```python
from build123d import *

# Parameters (mm, degrees)
SKETCH007_R  = 4
PAD003_DEPTH = 20
SKETCH001_R  = 4
PAD004_DEPTH = 32
PAD006_DEPTH = 4
PAD001_DEPTH = 4
SKETCH_R     = 4.1
PAD_DEPTH    = 80
PAD008_DEPTH = 10


with BuildPart() as rodhole01:
    # Sketch007 → Pad003 (new body)
    with BuildSketch(Plane.XZ.offset(15)):
        with Locations((30, 40)):
            Circle(SKETCH007_R)
        with Locations((-30, 40)):
            Circle(SKETCH007_R)
    extrude(amount=-PAD003_DEPTH)


with BuildPart() as rodhole02:
    # Sketch001 → Pad004 (new body)
    with BuildSketch(Plane.YZ.offset(16)):
        with Locations((-3.5, 70)):
            Circle(SKETCH001_R)
        with Locations((-3.5, 10)):
            Circle(SKETCH001_R)
    extrude(amount=-PAD004_DEPTH)


with BuildPart() as obj1:
    # Sketch002 → Pad006 (new body)
    with BuildSketch(Plane.YZ.offset(-11)):
        Polygon((3.9, 70), (0.2, 76.408588), (-7.2, 76.408588), (-10.9, 70), (-7.2, 63.591412), (0.2, 63.591412), align=None)
        Polygon((0.2, 3.591412), (3.9, 10), (0.2, 16.408588), (-7.2, 16.408588), (-10.9, 10), (-7.2, 3.591412), align=None)
    extrude(amount=-PAD006_DEPTH)


with BuildPart() as cutblock:
    # Sketch008 → Pad001 (new body)
    with BuildSketch(Plane.XZ.offset(-1)):
        Polygon((33.7, 33.591412), (37.4, 40), (33.7, 46.408588), (26.3, 46.408588), (22.6, 40), (26.3, 33.591412), align=None)
        Polygon((-26.3, 33.591412), (-22.6, 40), (-26.3, 46.408588), (-33.7, 46.408588), (-37.4, 40), (-33.7, 33.591412), align=None)
    extrude(amount=-PAD001_DEPTH)

    # Fusion001: union RodHole01, RodHole02, obj1
    add(rodhole01.part)
    add(rodhole02.part)
    add(obj1.part)


with BuildPart() as base:
    # Sketch → Pad (new body)
    with BuildSketch(Plane.XY):
        with BuildLine():
            Line((-15, 5), (-15, -15))
            Line((-15, -15), (15, -15))
            Line((15, -15), (15, 5))
            ThreePointArc((15, 5), (0, 15.432236), (-15, 5))
        make_face()
        with Locations((0, 5)):
            Circle(SKETCH_R, mode=Mode.SUBTRACT)
    extrude(amount=PAD_DEPTH)


with BuildPart() as cut:
    # Sketch010 → Pad008 (new body, symmetric)
    with BuildSketch(Plane.XZ.offset(5)):
        with BuildLine():
            ThreePointArc((-15, 20), (-20.986141, 27.270818), (-30.000033, 30))
            ThreePointArc((-30.000014, 50), (-40, 40.000009), (-30.000033, 30))
            ThreePointArc((-30.000014, 50), (-20.986133, 52.729187), (-15, 60))
            Line((-15, 60), (-15, 20))
        make_face()
        with BuildLine():
            ThreePointArc((15, 60), (20.986133, 52.729187), (30.000013, 50))
            ThreePointArc((30.000013, 30), (40, 40), (30.000013, 50))
            ThreePointArc((30.000013, 30), (20.986133, 27.270813), (15, 20))
            Line((15, 60), (15, 20))
        make_face()
    extrude(amount=PAD008_DEPTH, both=True)

    # Fusion: union Base
    add(base.part)

    # Cut: cut CutBlock
    add(cutblock.part, mode=Mode.SUBTRACT)


solid = cut.part
```
Can you work these out from the model? Positions are in its coordinate system, mm. A direction names the side the tool comes from. Give positions to 0.01 mm unless a question says otherwise; leave off trailing zeros. Write each loop counter-clockwise with the first axis right and the second up, starting at its lowest first coordinate (ties: lowest second). Pieces come first, ordered by that corner, then holes. Notation, with made-up numbers: (65.5, -38.5) - (117.5, -38.5) arc R32 cw to (117.5, -6.5) - close; hole circle Ø5 at (22.5, -1). An arc over 180 degrees is marked (long way). Write item = value, one per line. Start each with the question number.
1. On a 3-axis mill with a long thin cutter (end or side, diameter ignored), from which of +Z, -Z, +X, -X, +Y, -Y can I reach the whole of each face in a straight line? I mean faces 3 (the face through (-21.098, -4.86, 52.655)), 4 (the face through (-24.476, 2.972, 36.751)), 5 (the face through (-12.972, 2.076, 73.159)). Say none if no direction works.
2. Imagine slicing it at D-D (x = -28.5). Please give me the cut outline in (y, z).
3. Imagine slicing it at B-B (z = 41). Please give me the cut outline in (x, y), and give its area (3 significant figures).
4. For pin 1 (5 mm diameter, centred on y = 8.5, z = 25, fed in from +X); pin 2 (12 mm diameter, centred on x = -24, y = -5.5, fed in from -Z); pin 3 (8 mm diameter, centred on x = -17.5, z = 41.5, fed in from +Y), each with a flat end and sliding along its axis, tell me the tip position at first contact or that it passes through.
5. Imagine slicing it at C-C (y = -12). Please give me the cut outline in (x, z), and give its area (3 significant figures).
6. Imagine slicing it at A-A (y = -3.5). Count the separate pieces of the cut face and the enclosed holes in it, and give its area (3 significant figures).
7. Please list where these lines run through material, in increasing order: line 1 (Z direction, x = 3.5, y = -3.5); line 2 (Z direction, x = 30, y = -8); line 3 (X direction, y = -5, z = 42).
8. Thinking about a two-plate mould opening in Y: for faces 1 (the face through (-12.972, 2.024, 6.751)), 2 (the face through (-15, -9, 65)), which applies, released by +Y, released by -Y, zero draft, split by the parting line, or undercut?
Worked answers:
q1.face_3 = +Z, -X, +Y, -Y
q1.face_4 = +Y
q1.face_5 = -X
q2.outline = (-15, 29.93) - (5, 29.93) - (5, 33.59) - (1, 33.59) - (1, 36.29) - (-15, 36.29) - close; (-15, 43.71) - (1, 43.71) - (1, 46.41) - (5, 46.41) - (5, 50.07) - (-15, 50.07) - close
q3.outline = (-39.95, -15) - (-33.87, -15) - (-33.87, 1) - (-36.82, 1) - (-36.82, 5) - (-39.95, 5) - close; (-26.13, -15) - (26.13, -15) - (26.13, 1) - (23.18, 1) - (23.18, 5) - (15, 5) arc R16 ccw to (-15, 5) - (-23.18, 5) - (-23.18, 1) - (-26.13, 1) - close; (33.87, -15) - (39.95, -15) - (39.95, 5) - (36.82, 5) - (36.82, 1) - (33.87, 1) - close; hole circle Ø8.2 at (0, 5)
q3.area = 1,420 mm2
q4.pin_1 = 14.59
q4.pin_2 = 24.71
q4.pin_3 = 8.02
q5.outline = (-30, 30) arc R16.25 cw to (-15, 20) - (-15, 0) - (15, 0) - (15, 20) arc R16.25 cw to (30, 30) arc R10 ccw to (30, 50) arc R16.25 cw to (15, 60) - (15, 80) - (-15, 80) - (-15, 60) arc R16.25 cw to (-30, 50) arc R10 ccw to start; hole circle Ø8 at (-30, 40); hole circle Ø8 at (30, 40)
q5.area = 3,380 mm2
q6.separate_pieces = 3
q6.enclosed_holes = 2
q6.area = 2,860 mm2
q7.line_1 = 0 to 6, 14 to 66, 74 to 80
q7.line_2 = 30 to 36, 44 to 50
q7.line_3 = -39.8 to -33.46, -26.54 to 26.54, 33.46 to 39.8
q8.face_1 = undercut
q8.face_2 = zero draft
